from build123d import *

# Parameters (mm, degrees)
F2_W         = 30.1625
F2_H         = 19.05
F2_R         = 5.842
F2_R_2       = 1.8161
F3_DEPTH     = 2.54
F5_DEPTH     = 2.032
F7_DEPTH     = 6.35
F8_DEPTH     = 2.032
F9_DEPTH     = 2.032
F11_DEPTH    = 14.32025
F12_R        = 5.842
F13_DEPTH    = 12.41425
F14_R        = 2.54
F15_R        = 0.4064
F16_R        = 0.254
F17_T1_DEPTH = 18.2149387894
F18_T1_DEPTH = 29.845


# Not quite as in the source:
# - a fillet or chamfer that OpenCascade refuses, or shapes differently, is made with other operations: its cross-section is extruded or revolved along the edge and cut away or added


with BuildPart() as f3:
    # F2 (on Top) → F3 (new body)
    with BuildSketch(Plane.XY):
        with Locations((5.55625, 0)):
            Rectangle(F2_W, F2_H)
        Circle(F2_R, mode=Mode.SUBTRACT)
        Circle(F2_R)
        Circle(F2_R_2, mode=Mode.SUBTRACT)
    extrude(amount=F3_DEPTH)

    # F4 (on Front) → F5 (join, symmetric)
    with BuildSketch(Plane.XZ):
        with BuildLine():
            ThreePointArc((1.5351403895, 1.905), (-4.9973131459, 6.6442757011), (-7.493, 14.31925))
            Line((-7.493, 14.31925), (-9.525, 14.31925))
            Line((-9.525, 14.31925), (-9.525, 0))
            Line((-9.525, 0), (20.6375, 0))
            Line((20.6375, 0), (20.6375, 14.31925))
            Line((20.6375, 14.31925), (18.6055, 14.31925))
            ThreePointArc((18.6055, 14.31925), (16.1098131459, 6.6442757011), (9.5773596105, 1.905))
            Line((9.5773596105, 1.905), (1.5351403895, 1.905))
        make_face()
    extrude(amount=F5_DEPTH, both=True)

    # F6 (on face) → F7 (join)
    with BuildSketch(Plane.XZ.offset(2.032)):
        with BuildLine():
            Line((-3.175, 14.31925), (-9.525, 14.31925))
            Line((-9.525, 14.31925), (-9.525, 0))
            Line((-9.525, 0), (20.6375, 0))
            Line((20.6375, 0), (20.6375, 14.31925))
            Line((20.6375, 14.31925), (14.2875, 14.31925))
            ThreePointArc((14.2875, 14.31925), (5.55625, 5.588), (-3.175, 14.31925))
        make_face()
    extrude(amount=F7_DEPTH)

    # F4 (on Front) → F8 (cut, symmetric)
    with BuildSketch(Plane.XZ):
        with BuildLine():
            ThreePointArc((0.3585509899, 4.318), (-4.0776910817, 8.4687580722), (-5.715, 14.31925))
            Line((-5.715, 14.31925), (-7.493, 14.31925))
            ThreePointArc((-7.493, 14.31925), (-4.9973131459, 6.6442757011), (1.5351403895, 1.905))
            Line((1.5351403895, 1.905), (9.5773596105, 1.905))
            ThreePointArc((9.5773596105, 1.905), (16.1098131459, 6.6442757011), (18.6055, 14.31925))
            Line((18.6055, 14.31925), (16.8275, 14.31925))
            ThreePointArc((16.8275, 14.31925), (15.1901910817, 8.4687580722), (10.7539490101, 4.318))
            Line((10.7539490101, 4.318), (0.3585509899, 4.318))
        make_face()
    extrude(amount=F8_DEPTH, both=True, mode=Mode.SUBTRACT)

    # F4 (on Front) → F9 (join, through all)
    with BuildSketch(Plane.XZ):
        with BuildLine():
            ThreePointArc((14.2875, 14.31925), (5.55625, 5.588), (-3.175, 14.31925))
            Line((-3.175, 14.31925), (-5.715, 14.31925))
            ThreePointArc((-5.715, 14.31925), (-4.0776910817, 8.4687580722), (0.3585509899, 4.318))
            Line((0.3585509899, 4.318), (10.7539490101, 4.318))
            ThreePointArc((10.7539490101, 4.318), (15.1901910817, 8.4687580722), (16.8275, 14.31925))
            Line((16.8275, 14.31925), (14.2875, 14.31925))
        make_face()
    extrude(amount=F9_DEPTH)

    # F10: F3 across plane


with BuildPart() as f3_1:
    add(f3.part)
    add(f3.part.mirror(Plane.XZ))

    # F2 (on Top) → F11 (cut, through all)
    with BuildSketch(Plane.XY):
        Circle(F2_R_2)
    extrude(amount=F11_DEPTH, mode=Mode.SUBTRACT)

    # F12 (on face) → F13 (cut, through all)
    with BuildSketch(Plane.XY.offset(14.31925)):
        Circle(F12_R)
    extrude(amount=-F13_DEPTH, mode=Mode.SUBTRACT)

    # F14
    f14_edges = [f3_1.edges().sort_by_distance(p)[0] for p in [
        (20.6375, 9.525, 1.27),
        (-9.525, 9.525, 1.27),
        (20.6375, -9.525, 1.27),
        (-9.525, -9.525, 1.27),
    ]]
    fillet(f14_edges, radius=F14_R)

    # F15
    f15_edges = [f3_1.edges().sort_by_distance(p)[0] for p in [
        (5.55625, -8.382, 5.588),
        (5.55625, 8.382, 5.588),
    ]]
    fillet(f15_edges, radius=F15_R)

    # F16
    f16_edges = [f3_1.edges().sort_by_distance(p)[0] for p in [
        (-5.842, 0, 1.905),
    ]]
    fillet(f16_edges, radius=F16_R)

    # F17: fillet of radius 2.54 on 4 edges, made by hand

    # F17_s2 → F17_t1 (cut)
    with BuildSketch(Plane.XY.offset(2.54)):
        with BuildLine():
            ThreePointArc((-6.985, -8.382), (-8.7810512242, -7.6380512242), (-9.525, -5.842))
            Line((-9.525, -5.842), (-9.779, -5.842))
            ThreePointArc((-9.779, -5.842), (-9.779, -6.985), (-9.3184500445, -8.5217))
            Line((-9.3184500445, -8.5217), (-9.1063182222, -8.636))
            Line((-9.1063182222, -8.636), (-6.985, -8.636))
            Line((-6.985, -8.636), (-6.985, -8.382))
        make_face()
        with BuildLine():
            ThreePointArc((18.0975, -8.382), (19.8935512242, -7.6380512242), (20.6375, -5.842))
            Line((20.6375, -5.842), (20.8915, -5.842))
            ThreePointArc((20.8915, -5.842), (20.8915, -6.985), (20.4309500445, -8.5217))
            Line((20.4309500445, -8.5217), (20.2188182222, -8.636))
            Line((20.2188182222, -8.636), (18.0975, -8.636))
            Line((18.0975, -8.636), (18.0975, -8.382))
        make_face()
        with BuildLine():
            ThreePointArc((20.6375, 5.842), (19.8935512242, 7.6380512242), (18.0975, 8.382))
            Line((18.0975, 8.382), (18.0975, 8.636))
            Line((18.0975, 8.636), (20.2188182222, 8.636))
            Line((20.2188182222, 8.636), (20.4309500445, 8.5217))
            ThreePointArc((20.4309500445, 8.5217), (20.8915, 6.985), (20.8915, 5.842))
            Line((20.8915, 5.842), (20.6375, 5.842))
        make_face()
        with BuildLine():
            ThreePointArc((-6.985, 8.382), (-8.7810512242, 7.6380512242), (-9.525, 5.842))
            Line((-9.525, 5.842), (-9.779, 5.842))
            ThreePointArc((-9.779, 5.842), (-9.779, 6.985), (-9.3184500445, 8.5217))
            Line((-9.3184500445, 8.5217), (-9.1063182222, 8.636))
            Line((-9.1063182222, 8.636), (-6.985, 8.636))
            Line((-6.985, 8.636), (-6.985, 8.382))
        make_face()
    extrude(amount=F17_T1_DEPTH, mode=Mode.SUBTRACT)

    # F18: fillet of radius 3.175 on 2 edges, made by hand

    # F18_s2 → F18_t1 (cut)
    with BuildSketch(Plane.XZ.offset(-14.9225)):
        with BuildLine():
            ThreePointArc((17.4625, 0), (19.7075640303, 0.9299359697), (20.6375, 3.175))
            Line((20.6375, 3.175), (20.6375, 0))
            Line((20.6375, 0), (17.4625, 0))
        make_face()
        with BuildLine():
            ThreePointArc((-9.525, 3.175), (-8.5950640303, 0.9299359697), (-6.35, 0))
            Line((-6.35, 0), (-9.525, 0))
            Line((-9.525, 0), (-9.525, 3.175))
        make_face()
    extrude(amount=F18_T1_DEPTH, mode=Mode.SUBTRACT)


solid = f3_1.part
Verification items for the finished model (mm, model axes). A direction names the side the tool comes from. Coordinates: 2 decimals unless noted, no trailing zeros. Order: outer loops, then holes, each group sorted by start corner. A loop starts at its lowest first (then second) coordinate and runs counter-clockwise, first axis right, second up.
Item 1: Material ranges on L1, parallel to Y at x = 0, z = 6.25; L2, parallel to Y at x = 0, z = 0.9 (3 decimals); L3, parallel to X at y = 0, z = 7.25 (1 decimal), recorded low to high.
Filled in:
L1: y = -8.38 to -5.84, 5.84 to 8.38
L2: y = -9.525 to -1.816, 1.816 to 9.525
L3: x = -9.5 to -5.8, 10.7 to 14.3, 16.5 to 20.6
Item 2: Section check A-A, the plane y = 0. Give the number of separate pieces and of enclosed holes in the cut face, then the cut area to 3 significant figures.
Filled in:
separate pieces: 3
enclosed holes: 0
area: 175 mm2
Item 3: Section check B-B, the plane z = 1. Enter the section's corners in (x, y) (1 decimal), then the cut area to 3 significant figures.
Filled in:
outline: (-8.7, -8.9) arc R2.5 ccw to (-7, -9.5) - (18.1, -9.5) arc R2.5 ccw to (19.8, -8.9) - (19.8, 8.9) arc R2.5 ccw to (18.1, 9.5) - (-7, 9.5) arc R2.5 ccw to (-8.7, 8.9) - close; hole circle Ø3.6 at (0, 0)
area: 530 mm2
Item 4: Access from +Z, -Z, +X, -X, +Y, -Y to the whole of each face (thin tool, end or side, straight path). Record for faces 1 (the face through (-5.836, 0.257, 6.973)), 2 (the face through (-6, -2.032, 12)), 3 (the face through (5, 0, 0)), 4 (the face through (5, -8.382, 5)).
Filled in:
face 1: +Z
face 2: none
face 3: -Z, +X, -X, +Y, -Y
face 4: +Z, +X, -X, -Y
Item 5: Depth check by flat-ended pin: pin 1 (3.5 mm diameter, centred on x = 11, z = 7, fed in from +Y); pin 2 (4 mm diameter, centred on x = 16.5, z = 6, fed in from -Y); pin 3 (0.9 mm diameter, centred on x = 13, y = 8.5, fed in from +Z). Enter the tip coordinate at first touch or a pass-through.
Filled in:
pin 1: stops at y = 8.38
pin 2: stops at y = -8.38
pin 3: stops at z = 10.21
Item 6: Release check for a two-part mould opening along Z. For faces 5 (the face through (19.87, -7.66, 8.35)), 6 (the face through (5, -9, 2.54)), 7 (the face through (8, 0, 4.318)) record: +Z half, -Z half, draft (parallel to the pull), parting line (faces both ways), or undercut.
Filled in:
face 5: draft
face 6: +Z half
face 7: undercut
